Check sheet for the modelled part. Datum: model origin and axes. Units: mm. Coordinates: 2 decimals unless noted, no trailing zeros. Loops run counter-clockwise (first coordinate to the right, second up) from the corner with the lowest first, then second, coordinate; pieces in that order, holes last.
from build123d import *

# Parameters (mm, degrees)
BOSS_EXTRUDE1_DEPTH = 7
SKETCH3_R           = 2.5
CUT_EXTRUDE1_DEPTH  = 14


with BuildPart() as part:
    # Sketch2 → Boss-Extrude1 (new body)
    with BuildSketch(Plane(origin=(0, 0, 0), x_dir=(1, 0, 0), z_dir=(0, 1, 0))):
        with BuildLine():
            Line((-2.748329621, 10.673719376), (23.251670379, 10.673719376))
            Line((23.251670379, 10.673719376), (23.251670379, -3.326280624))
            Line((23.251670379, -3.326280624), (-2.748329621, -3.326280624))
            ThreePointArc((-2.748329621, -3.326280624), (-5.576756746, -2.154707748), (-6.748329621, 0.673719376))
            Line((-6.748329621, 0.673719376), (-6.748329621, 6.673719376))
            ThreePointArc((-6.748329621, 6.673719376), (-5.576756746, 9.502146501), (-2.748329621, 10.673719376))
        make_face()
    extrude(amount=BOSS_EXTRUDE1_DEPTH)

    # Sketch3 → Cut-Extrude1 (cut)
    with BuildSketch(Plane.XY.offset(3.326280624)):
        with Locations((-2.748329621, 3.5)):
            Circle(SKETCH3_R)
    extrude(amount=-CUT_EXTRUDE1_DEPTH, mode=Mode.SUBTRACT)


solid = part.part
(1) Section check C-C, the plane y = 3.5. Enter the section's corners in (x, z), plus the area to 3 significant figures.
(2) Section check B-B, the plane y = 5.5. Enter the section's corners in (x, z).
(3) Section check A-A, the plane z = -2.25. Enter the section's corners in (x, y), plus the area to 3 significant figures.
(4) Section check D-D, the plane z = 1. Enter the section's corners in (x, y), plus the area to 3 significant figures.
(5) Gauge pin test, flat end, axial feed: P1, Ø8, axis at x = 12.5, z = 1, coming from the -Y side. Record the tip position at first contact, or that the pin passes through.
(6) Scan lines: line 1 along X through (y, z) = (3.5, -4.25); line 2 along X through (y, z) = (5.5, -1.5); line 3 along Y through (x, z) = (-4, -9). Record each from-to range of solid material in increasing order.
(7) Draft check along X on faces 1 (the face through (-6, 3.451, 1.656)), 2 (the face through (10, 3, -10.674)), 3 (the face through (-0.364, 4.251, -3.576)). Enter one of: pulls with the +X half, pulls with the -X half, needs draft (parallel to the pull), parting line crosses it, or undercut.
Determined:
1. outline: (-6.75, -6.67) arc R4 ccw to (-5.25, -9.8) - (-5.25, 2.45) arc R4 ccw to (-6.75, -0.67) - close; (-0.25, -10.67) - (23.25, -10.67) - (23.25, 3.33) - (-0.25, 3.33) - close
1. area: 345 mm2
2. outline: (-6.75, -6.67) arc R4 ccw to (-4.25, -10.38) - (-4.25, 3.03) arc R4 ccw to (-6.75, -0.67) - close; (-1.25, -10.67) - (23.25, -10.67) - (23.25, 3.33) - (-1.25, 3.33) - close
3. outline: (-6.75, 0) - (23.25, 0) - (23.25, 7) - (-6.75, 7) - close; hole circle Ø5 at (-2.75, 3.5)
3. area: 190 mm2
4. outline: (-6.38, 0) - (23.25, 0) - (23.25, 7) - (-6.38, 7) - close; hole circle Ø5 at (-2.75, 3.5)
4. area: 188 mm2
5. P1: stops at y = 0
6. line 1: x = -6.75 to -5.25, -0.25 to 23.25
6. line 2: x = -6.75 to -4.25, -1.25 to 23.25
6. line 3: y = 0 to 1.34, 5.66 to 7
7. face 1: pulls with the -X half
7. face 2: needs draft
7. face 3: undercut
